```python
from build123d import *

# Parameters (mm, degrees)
SKETCH_1_R          = 2.55
EXTRUDE_1_DEPTH     = 4.5
SKETCH_2_W          = 6
SKETCH_2_H          = 20
EXTRUDE_2_DEPTH     = 29
SKETCH_5_W          = 33.5
SKETCH_5_H          = 4.5
EXTRUDE_4_DEPTH     = 13
SKETCH_6_R          = 1.5
CUT_EXTRUDE_1_DEPTH = 13
SKETCH_8_W          = 6
SKETCH_8_H          = 20
EXTRUDE_5_DEPTH     = 10
SKETCH_11_W         = 6
SKETCH_11_H         = 43.5
EXTRUDE_7_DEPTH     = 30
SKETCH_17_W         = 6
SKETCH_17_H         = 43.5
CUT_EXTRUDE_3_DEPTH = 14
SKETCH_18_W         = 6
SKETCH_18_H         = 16.247997213
EXTRUDE_12_DEPTH    = 10
SKETCH_20_W         = 15
SKETCH_20_H         = 4.5
EXTRUDE_13_DEPTH    = 15
SKETCH_22_R         = 1.5
CUT_EXTRUDE_5_DEPTH = 15
SKETCH_23_W         = 13
SKETCH_23_H         = 33.5
CUT_EXTRUDE_6_DEPTH = 15
SKETCH_24_R         = 1.5
CUT_EXTRUDE_7_DEPTH = 15


with BuildPart() as part:
    # 草图1 → 凸台-拉伸1 (new body)
    with BuildSketch(Plane.XY):
        Polygon((-27.5, -10), (21.5, -10), (21.5, 10), (-27.5, 10), (-33.5, 10), (-33.5, -10), align=None)
        with Locations((-15.85, 0)):
            Circle(SKETCH_1_R, mode=Mode.SUBTRACT)
        with Locations((15.85, 0)):
            Circle(SKETCH_1_R, mode=Mode.SUBTRACT)
        with BuildLine():
            Line((-8.144701861, 2.212014563), (8.144701861, 2.212014563))
            ThreePointArc((8.144701861, 2.212014563), (10.356716424, 0), (8.144701861, -2.212014563))
            Line((8.144701861, -2.212014563), (-8.144701861, -2.212014563))
            ThreePointArc((-8.144701861, -2.212014563), (-10.356716424, 0), (-8.144701861, 2.212014563))
        make_face(mode=Mode.SUBTRACT)
    extrude_1 = extrude(amount=EXTRUDE_1_DEPTH)

    # 草图2 → 凸台-拉伸2 (add)
    with BuildSketch(Plane.XY.offset(4.5)):
        with Locations((-30.5, 0)):
            Rectangle(SKETCH_2_W, SKETCH_2_H)
    extrude(amount=EXTRUDE_2_DEPTH)

    # 草图5 → 凸台-拉伸4 (add)
    with BuildSketch(Plane.ZY.offset(33.5)):
        with Locations((16.75, -7.75)):
            Rectangle(SKETCH_5_W, SKETCH_5_H)
        with Locations((16.75, 7.25)):
            Rectangle(SKETCH_5_W, SKETCH_5_H)
    extrude(amount=EXTRUDE_4_DEPTH)

    # 草图6 → 切除-拉伸1 (cut)
    with BuildSketch(Plane.XZ.offset(10)):
        with Locations((-39.2, 1.6)):
            Circle(SKETCH_6_R)
        with Locations((-39.2, 10.6)):
            Circle(SKETCH_6_R)
    extrude(amount=-CUT_EXTRUDE_1_DEPTH, mode=Mode.SUBTRACT)

    # 草图8 → 凸台-拉伸5 (add)
    with BuildSketch(Plane(origin=(0, 0, 0), x_dir=(-1, 0, 0), z_dir=(0, 0, -1))):
        with Locations((30.5, 0)):
            Rectangle(SKETCH_8_W, SKETCH_8_H)
    extrude(amount=EXTRUDE_5_DEPTH)

    # 草图11 → 凸台-拉伸7 (add)
    with BuildSketch(Plane(origin=(0, 10, 0), x_dir=(1, 0, 0), z_dir=(0, 1, 0))):
        with Locations((-30.5, -11.75)):
            Rectangle(SKETCH_11_W, SKETCH_11_H)
    extrude(amount=EXTRUDE_7_DEPTH)

    # 草图17 → 切除-拉伸3 (cut)
    with BuildSketch(Plane(origin=(0, 40, 0), x_dir=(1, 0, 0), z_dir=(0, 1, 0))):
        with Locations((-30.5, -11.75)):
            Rectangle(SKETCH_17_W, SKETCH_17_H)
    extrude(amount=-CUT_EXTRUDE_3_DEPTH, mode=Mode.SUBTRACT)

    # 草图18 → 凸台-拉伸12 (add)
    with BuildSketch(Plane(origin=(0, 26, 0), x_dir=(1, 0, 0), z_dir=(0, 1, 0))):
        with Locations((-30.5, -10.74216301)):
            Rectangle(SKETCH_18_W, SKETCH_18_H)
    extrude(amount=EXTRUDE_12_DEPTH)

    # 镜向1: 凸台-拉伸1 across plane
    add(extrude_1.mirror(Plane.ZX.offset(10)))

    # 草图20 → 凸台-拉伸13 (add)
    with BuildSketch(Plane.ZY.offset(33.5)):
        with Locations((-7.5, 7.25)):
            Rectangle(SKETCH_20_W, SKETCH_20_H)
    extrude(amount=EXTRUDE_13_DEPTH)

    # 草图22 → 切除-拉伸5 (cut)
    with BuildSketch(Plane.XZ.offset(-5)):
        with Locations((-39.2, 10.6)):
            Circle(SKETCH_22_R)
        with Locations((-39.2, 1.6)):
            Circle(SKETCH_22_R)
    extrude(amount=-CUT_EXTRUDE_5_DEPTH, mode=Mode.SUBTRACT)

    # 草图23 → 切除-拉伸6 (cut)
    with BuildSketch(Plane.XZ.offset(10)):
        with Locations((-40, 16.75)):
            Rectangle(SKETCH_23_W, SKETCH_23_H)
    extrude(amount=-CUT_EXTRUDE_6_DEPTH, mode=Mode.SUBTRACT)

    # 草图24 → 切除-拉伸7 (cut)
    with BuildSketch(Plane.XZ.offset(-5)):
        with Locations(Location((-39.19836294, -7.4, 0), (0, 0, 270))):
            Circle(SKETCH_24_R)
    extrude(amount=-CUT_EXTRUDE_7_DEPTH, mode=Mode.SUBTRACT)


solid = part.part
```
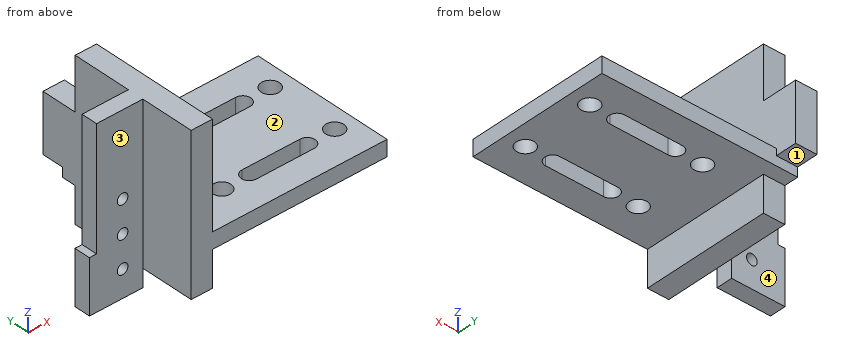
Verification items for the finished model (mm, model axes). Face numbers are marked on the shaded views. A direction names the side the tool comes from. Coordinates: 2 decimals unless noted, no trailing zeros. Loops run counter-clockwise (first coordinate to the right, second up) from the corner with the lowest first, then second, coordinate; pieces in that order, holes last. Notation, with made-up numbers: (46.25, 53.25) -> (75.25, 53.25) arc R22 cw to (75.25, 85.25) -> close; hole circle Ø5 at (79.25, 86.25). An arc over 180 degrees is marked (long way). Put each result on its own line as item: value.
1. Section check A-A, the plane z = 1.6. Record the boundary of the cut face in (x, y).
Result set:
outline: (-46.5, 5) -> (-40.7, 5) -> (-40.7, 9.5) -> (-46.5, 9.5) -> close; (-37.7, 5) -> (-33.5, 5) -> (-33.5, -10) -> (21.5, -10) -> (21.5, 30) -> (-33.5, 30) -> (-33.5, 9.5) -> (-37.7, 9.5) -> close; hole circle Ø5.1 at (-15.85, 0); hole circle Ø5.1 at (-15.85, 20); hole (-8.14, -2.21) -> (8.14, -2.21) arc R2.21 ccw to (8.14, 2.21) -> (-8.14, 2.21) arc R2.21 ccw to start; hole (-8.14, 17.79) -> (8.14, 17.79) arc R2.21 ccw to (8.14, 22.21) -> (-8.14, 22.21) arc R2.21 ccw to start; hole circle Ø5.1 at (15.85, 0); hole circle Ø5.1 at (15.85, 20)
2. Tool access check on the marked faces 1, 2, 3 and 4. Record the directions out of +Z, -Z, +X, -X, +Y, -Y that give a thin tool (end or side, any length) a straight path to the whole face; none if there is none.
Result set:
face 1: -Z, +X, -X, +Y
face 2: +Z, +X, +Y, -Y
face 3: +Z, -Z, -X, -Y
face 4: +Z, -Z, -X, +Y
3. Thickness scan on line 1 (Y direction, x = 15.85, z = 2.75); line 2 (Z direction, x = -39.2, y = 6.85); line 3 (X direction, y = 20, z = 3). Record the ranges inside material, lowest first.
Result set:
line 1: y = -10 to -2.55, 2.55 to 17.45, 22.55 to 30
line 2: z = -15 to -8.9, -5.9 to 0.1, 3.1 to 9.1, 12.1 to 33.5
line 3: x = -33.5 to -18.4, -13.3 to -10.36, 10.36 to 13.3, 18.4 to 21.5
4. Section check C-C, the plane z = 10.6. Record the boundary of the cut face in (x, y), then the cut area to 3 significant figures.
Result set:
outline: (-46.5, 5) -> (-40.7, 5) -> (-40.7, 9.5) -> (-46.5, 9.5) -> close; (-37.7, 5) -> (-33.5, 5) -> (-33.5, -10) -> (-27.5, -10) -> (-27.5, 36) -> (-33.5, 36) -> (-33.5, 9.5) -> (-37.7, 9.5) -> close
area: 321 mm^2
5. Gauge pin test, flat ends, axial feed: P1, Ø2, axis at x = -3.5, z = 3, coming from the +Y side; P2, Ø12, axis at x = -6, y = -3.5, coming from the -Z side; P3, Ø12, axis at x = -7.5, y = 16.5, coming from the +Z side; P4, Ø1.8, axis at x = -39.2, z = 1.6, coming from the +Y side. Record the tip position at first contact, or that the pin passes through.
Result set:
P1: stops at y = 30
P2: stops at z = 0
P3: stops at z = 4.5
P4: passes through
6. Section check D-D, the plane y = 20. Record the boundary of the cut face in (x, z).
Result set:
outline: (-33.5, -10) -> (-27.5, -10) -> (-27.5, 0) -> (-18.4, 0) -> (-18.4, 4.5) -> (-27.5, 4.5) -> (-27.5, 33.5) -> (-33.5, 33.5) -> close; (-13.3, 0) -> (-10.36, 0) -> (-10.36, 4.5) -> (-13.3, 4.5) -> close; (10.36, 0) -> (13.3, 0) -> (13.3, 4.5) -> (10.36, 4.5) -> close; (18.4, 0) -> (21.5, 0) -> (21.5, 4.5) -> (18.4, 4.5) -> close
7. Section check B-B, the plane x = 15.85. Record the boundary of the cut face in (y, z), then the cut area to 3 significant figures.
Result set:
outline: (-10, 0) -> (-2.55, 0) -> (-2.55, 4.5) -> (-10, 4.5) -> close; (2.55, 0) -> (17.45, 0) -> (17.45, 4.5) -> (2.55, 4.5) -> close; (22.55, 0) -> (30, 0) -> (30, 4.5) -> (22.55, 4.5) -> close
area: 134 mm^2
